The figure shows three views and two pictorial views of one solid part (mm, origin at its lowest corner). Answer the questions. Coordinates: 2 decimals unless noted, no trailing zeros. Order: outer loops, then holes, each group sorted by start corner. A loop starts at its lowest first (then second) coordinate and runs counter-clockwise, first axis right, second up.
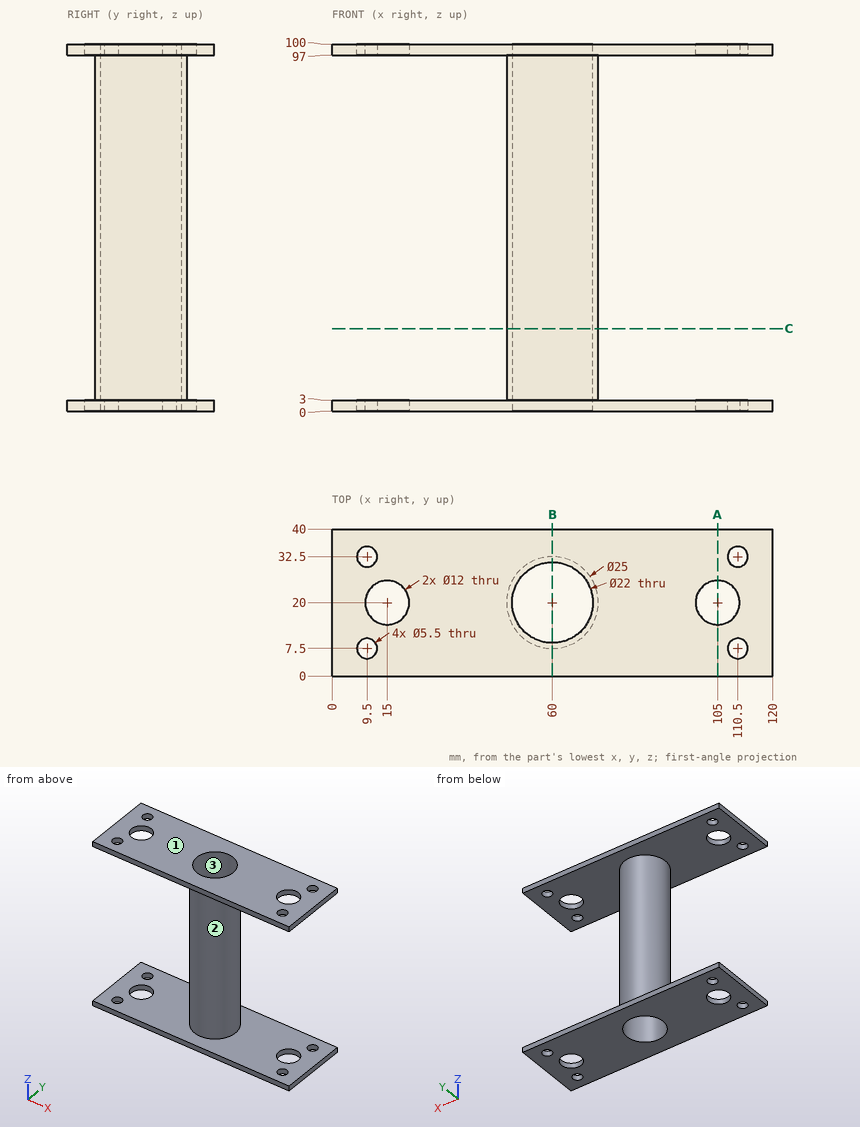
1) Each of these flat-tipped pins is pushed along its axis until it touches: P1, Ø4, axis at y = 18, z = 65, coming from the +X side; P2, Ø6, axis at y = 31, z = 24, coming from the +X side; P3, Ø1, axis at y = 8.5, z = 14.5, coming from the -X side. Where does it stop, or does it pass through?
2) A cutting plane is placed at C-C, the plane z = 22.5. Write down the section's boundary in (x, y), plus the area to 3 significant figures.
3) A cutting plane is placed at A-A, the plane x = 105. Write down the section's boundary in (y, z), plus the area to 3 significant figures.
4) A cutting plane is placed at B-B, the plane x = 60. Write down the section's boundary in (y, z).
5) The mould has two halves that part along Y. Classify the marked faces 1, 2 and 3: released by +Y, released by -Y, zero draft, split by the parting line, or undercut.
6) Straight lines are drawn through the part: probe 1 along Z at (x, y) = (73.5, 17); probe 2 along Y at (x, z) = (110.5, 2); probe 3 along X at (y, z) = (21.5, 66.5). For each, find the intervals that lie inside material, in ascending order.
Working result:
1. P1: stops at x = 72.5
1. P2: stops at x = 69.6
1. P3: stops at x = 54.06
2. outline: circle Ø25 at (60, 20); hole circle Ø22 at (60, 20)
2. area: 111 mm2
3. outline: (0, 0) - (14, 0) - (14, 3) - (0, 3) - close; (0, 97) - (14, 97) - (14, 100) - (0, 100) - close; (26, 0) - (40, 0) - (40, 3) - (26, 3) - close; (26, 97) - (40, 97) - (40, 100) - (26, 100) - close
3. area: 168 mm2
4. outline: (0, 0) - (9, 0) - (9, 100) - (0, 100) - (0, 97) - (7.5, 97) - (7.5, 3) - (0, 3) - close; (31, 0) - (40, 0) - (40, 3) - (32.5, 3) - (32.5, 97) - (40, 97) - (40, 100) - (31, 100) - close
5. face 1: zero draft
5. face 2: split by the parting line
5. face 3: undercut
6. probe 1: z = 0 to 3, 97 to 100
6. probe 2: y = 0 to 4.75, 10.25 to 17.6, 22.4 to 29.75, 35.25 to 40
6. probe 3: x = 47.59 to 49.1, 70.9 to 72.41
